Solid Edge part; units mm, degrees
sketch "Sketch1" plane through (0, 0, 0) normal (0, -1, 0) x (1, 0, 0)
  line L0 (3, 0) -> (3, 8)
  line L1 (3, 8) -> (0, 8)
  line L2 (0, 8) -> (0, 0)
  dimension "D1" = 3
revolve "RevolvedProtrusion1" add sketch "Sketch1" angle 360 about axis through (0, 0, 0) along (1, 0, 0)
sketch "Sketch2" plane through (3, 0, 0) normal (1, 0, 0) x (0, 1, 0)
  line L0 (-1.5411, 2.125) -> (1.5411, 2.125)
  arc A0 (1.5411, 2.125) -> (-1.5411, 2.125) centre (0, 0) cw
extrude "Protrusion1" add sketch "Sketch2" along normal blind 3
chamfer "Fase_2" distance 0.1 angle 45 2 edges at (6, 0, -2.625) (6, 0, 2.125)
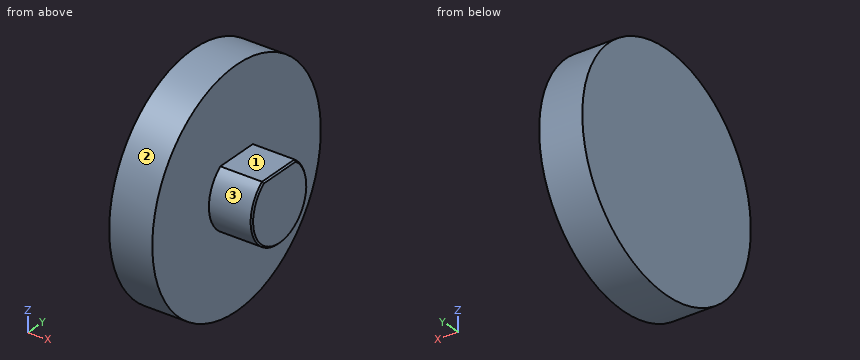
Source: CAD feature listing. Evaluate the final solid. Frame: model axes, mm. Face numbers are marked on the shaded views. A direction names the side the tool comes from. Coordinates: 2 decimals unless noted, no trailing zeros. Loops run counter-clockwise (first coordinate to the right, second up) from the corner with the lowest first, then second, coordinate; pieces in that order, holes last. Notation, with made-up numbers: (73.5, -33.75) - (80.5, -33.75) arc R9 cw to (80.5, -17.75) - close; hole circle Ø11 at (67.25, -10). An arc over 180 degrees is marked (long way). Answer as CSV lines item,"result".
1. Section B-B (y = 0). Return loops of the section in (x, z) (3 decimals).
Established:
outline,"(0, -8) - (3, -8) - (3, -2.625) - (5.9, -2.625) - (6, -2.525) - (6, 2.025) - (5.9, 2.125) - (3, 2.125) - (3, 8) - (0, 8) - close"
2. Ray query, line 1 (X direction, y = -3.25, z = -4.75); line 2 (Z direction, x = 0.9, y = -0.75); line 3 (Z direction, x = 0.3, y = -2.75). Return the intervals inside material, ascending.
Established:
line 1,"x = 0 to 3"
line 2,"z = -7.96 to 7.96"
line 3,"z = -7.51 to 7.51"
3. Section A-A (z = 0). Return loops of the section in (x, y) (3 decimals), then the cut area to 3 significant figures.
Established:
outline,"(0, -8) - (3, -8) - (3, -2.625) - (5.9, -2.625) - (6, -2.525) - (6, 2.525) - (5.9, 2.625) - (3, 2.625) - (3, 8) - (0, 8) - close"
area,"63.7 mm2"
4. Section C-C (x = 4.7). Return loops of the section in (y, z) (3 decimals), then the cut area to 3 significant figures.
Established:
outline,"(-1.541, 2.125) arc R2.625 ccw (long way) to (1.541, 2.125) - close"
area,"20.6 mm2"
5. Section D-D (x = 1.1). Return loops of the section in (y, z), then the cut area to 3 significant figures.
Established:
outline,"circle Ø16 at (0, 0)"
area,"201 mm2"
6. Contact query for flat-ended pins moving along their axis: pin 1 (2 mm diameter, centred on x = 1, z = -1.5, fed in from +Y); pin 2 (4 mm diameter, centred on y = 2.5, z = 3.5, fed in from +X); pin 3 (3 mm diameter, centred on x = 2, z = -4.5, fed in from -Y); pin 4 (1.5 mm diameter, centred on x = 5, y = -0.5, fed in from +Z) (3 decimals). Output: stop coordinate, or through.
Established:
pin 1,"stops at y = 7.98"
pin 2,"stops at x = 6"
pin 3,"stops at y = -7.42"
pin 4,"stops at z = 2.125"
7. Reachability of the marked faces 1, 2 and 3 from +Z, -Z, +X, -X, +Y, -Y: full face, straight path, thin tool, end or side. Return the list, or none.
Established:
face 1,"+Z, +X, +Y, -Y"
face 2,"+X, -X"
face 3,"+X"
